Geometry: final body of the model. Coordinates: model frame, mm. A direction names the side the tool comes from. Round coordinates to 2 decimals unless told otherwise and drop trailing zeros. Loops run counter-clockwise (first coordinate to the right, second up) from the corner with the lowest first, then second, coordinate; pieces in that order, holes last. Notation, with made-up numbers: (-37.75, 76) - (9.25, 76) arc R23 ccw to (9.25, 85) - close; hole circle Ø9 at (11, 16). An arc over 180 degrees is marked (long way). Use CSV: the item, a comma, the result in double quotes.
from build123d import *

# Parameters (mm, degrees)
SKETCH1_R                              = 175
BOSS_EXTRUDE1_DEPTH                    = 30
CSK_FOR_M10_SFHCS1_D                   = 11
CSK_FOR_M10_SFHCS1_CSINK_D             = 22.4
CSK_FOR_M10_SFHCS1_CSINK_ANGLE         = 90
F_6_0MM_DOWEL_HOLE1_D                  = 6
CUT_EXTRUDE2_DEPTH                     = 10
TAP_DRILL_FOR_M12X1_75_TAP1_AT_2_COUNT = 2
TAP_DRILL_FOR_M12X1_75_TAP1_AT_2_PITCH = 116
TAP_DRILL_FOR_M12X1_75_TAP1_AT_3_COUNT = 2
TAP_DRILL_FOR_M12X1_75_TAP1_AT_3_PITCH = 257.596583828
TAP_DRILL_FOR_M12X1_75_TAP1_AT_4_COUNT = 2
TAP_DRILL_FOR_M12X1_75_TAP1_AT_4_PITCH = 230


with BuildPart() as part:
    # Sketch1 → Boss-Extrude1 (new body)
    with BuildSketch(Plane(origin=(0, 0, 0), x_dir=(1, 0, 0), z_dir=(0, 1, 0))):
        Circle(SKETCH1_R)
    extrude(amount=BOSS_EXTRUDE1_DEPTH)

    # CSK for M10 SFHCS1 (through all)
    with Locations(Plane(origin=(0, 30, 0), x_dir=(1, 0, 0), z_dir=(0, 1, 0))):
        with Locations((-150, 0), (0, -150), (150, 0), (0, 150)):
            CounterSinkHole(CSK_FOR_M10_SFHCS1_D / 2, CSK_FOR_M10_SFHCS1_CSINK_D / 2, counter_sink_angle=CSK_FOR_M10_SFHCS1_CSINK_ANGLE)

    # Ø6.0mm Dowel Hole1 (through all)
    with Locations(Plane(origin=(0, 30, 0), x_dir=(1, 0, 0), z_dir=(0, 1, 0))):
        with Locations((-97.227182413, -97.227182413), (97.227182413, -97.227182413), (97.227182413, 97.227182413), (-97.227182413, 97.227182413)):
            Hole(F_6_0MM_DOWEL_HOLE1_D / 2)

    # Sketch14 → Cut-Extrude2 (cut)
    with BuildSketch(Plane(origin=(0, 30, 0), x_dir=(1, 0, 0), z_dir=(0, 1, 0))):
        with BuildLine():
            Line((-74, -40), (74, -40))
            ThreePointArc((74, -40), (78.242640687, -41.757359313), (80, -46))
            Line((80, -46), (80, -84))
            ThreePointArc((80, -84), (78.242640687, -88.242640687), (74, -90))
            Line((74, -90), (-74, -90))
            ThreePointArc((-74, -90), (-78.242640687, -88.242640687), (-80, -84))
            Line((-80, -84), (-80, -46))
            ThreePointArc((-80, -46), (-78.242640687, -41.757359313), (-74, -40))
        make_face()
        with BuildLine():
            Line((80, 46), (80, 84))
            ThreePointArc((80, 84), (78.242640687, 88.242640687), (74, 90))
            Line((74, 90), (-74, 90))
            ThreePointArc((-74, 90), (-78.242640687, 88.242640687), (-80, 84))
            Line((-80, 84), (-80, 46))
            ThreePointArc((-80, 46), (-78.242640687, 41.757359313), (-74, 40))
            Line((-74, 40), (74, 40))
            ThreePointArc((74, 40), (78.242640687, 41.757359313), (80, 46))
        make_face()
    extrude(amount=-CUT_EXTRUDE2_DEPTH, mode=Mode.SUBTRACT)

    # Sketch21 → Tap Drill for M12x1.75 Tap1 (revolve, cut)
    with BuildSketch(Plane(origin=(-58, 30, -115), x_dir=(0, 0, 1), z_dir=(1, 0, 0))):
        Polygon((0, 0), (0, 30), (12.5, 30), (5.1, 19.43170475), (5.1, 0), align=None)
    tap_drill_for_m12x1_75_tap1 = revolve(axis=Axis((-58, 36.35, -115), (0, -1, 0)), mode=Mode.SUBTRACT)

    # Tap Drill for M12x1.75 Tap1 at 2: Tap Drill for M12x1.75 Tap1 ×2
    with Locations(*[(i * TAP_DRILL_FOR_M12X1_75_TAP1_AT_2_PITCH, 0, 0) for i in range(1, TAP_DRILL_FOR_M12X1_75_TAP1_AT_2_COUNT)]):
        add(tap_drill_for_m12x1_75_tap1, mode=Mode.SUBTRACT)

    # Tap Drill for M12x1.75 Tap1 at 3: Tap Drill for M12x1.75 Tap1 ×2
    with Locations(*[Vector(0.450316531, 0, 0.892868984) * (i * TAP_DRILL_FOR_M12X1_75_TAP1_AT_3_PITCH) for i in range(1, TAP_DRILL_FOR_M12X1_75_TAP1_AT_3_COUNT)]):
        add(tap_drill_for_m12x1_75_tap1, mode=Mode.SUBTRACT)

    # Tap Drill for M12x1.75 Tap1 at 4: Tap Drill for M12x1.75 Tap1 ×2
    with Locations(*[(0, 0, i * TAP_DRILL_FOR_M12X1_75_TAP1_AT_4_PITCH) for i in range(1, TAP_DRILL_FOR_M12X1_75_TAP1_AT_4_COUNT)]):
        add(tap_drill_for_m12x1_75_tap1, mode=Mode.SUBTRACT)


solid = part.part
Item 1: Section A-A on x = 0. Return the cut outline in (y, z), plus the area to 4 significant figures.
Final values:
outline,"(0, -175) - (30, -175) - (30, -161.2) - (24.3, -155.5) - (0, -155.5) - close; (0, -144.5) - (24.3, -144.5) - (30, -138.8) - (30, -90) - (20, -90) - (20, -40) - (30, -40) - (30, 40) - (20, 40) - (20, 90) - (30, 90) - (30, 138.8) - (24.3, 144.5) - (0, 144.5) - close; (0, 155.5) - (24.3, 155.5) - (30, 161.2) - (30, 175) - (0, 175) - close"
area,"8,775 mm²"
Item 2: Pin query (flat end, axial travel): P1, Ø3, axis at x = -17.5, y = 26, coming from the -Z side; P2, Ø8, axis at x = -97.23, z = 97.23, coming from the -Y side; P3, Ø13.5, axis at x = 58, z = -115, coming from the -Y side; P4, Ø17.5, axis at x = 0, z = -150, coming from the +Y side. Return the tip coordinate at first contact, or that it passes through.
Final values:
P1,"stops at z = -174.27"
P2,"stops at y = 0"
P3,"stops at y = 8.21"
P4,"stops at y = 27.55"
Item 3: Mould query, pull axis X, two halves, no side actions, for faces 3 (the cylindrical face through (-128.982, 14.79, -118.273)), 4 (the flat face through (-2, 0, -2)), 5 (the cylindrical face through (-61.4, 20.4, 111.2)). Classes: released by +X, released by -X, zero draft, split by the parting line, or undercut.
Final values:
face 3,"split by the parting line"
face 4,"zero draft"
face 5,"undercut"
Item 4: Material intervals for line 1 (Z direction, x = -61, y = 6); line 2 (Z direction, x = -58, y = 21.25); line 3 (Z direction, x = -58, y = 17.5), sorted ascending.
Final values:
line 1,"z = -164.02 to -122.74, -107.26 to 107.26, 122.74 to 164.02"
line 2,"z = -165.11 to -120.1, -109.9 to -90, -40 to 40, 90 to 109.9, 120.1 to 165.11"
line 3,"z = -165.11 to -120.1, -109.9 to 109.9, 120.1 to 165.11"
Item 5: Section C-C on z = 150. Return the cut outline in (x, y), plus the area to 3 significant figures.
Final values:
outline,"(-90.14, 0) - (-5.5, 0) - (-5.5, 24.3) - (-11.2, 30) - (-90.14, 30) - close; (5.5, 0) - (90.14, 0) - (90.14, 30) - (11.2, 30) - (5.5, 24.3) - close"
area,"5,050 mm²"
Item 6: Section B-B on z = 0. Return the cut outline in (x, y), plus the area to 4 significant figures.
Final values:
outline,"(-175, 0) - (-155.5, 0) - (-155.5, 24.3) - (-161.2, 30) - (-175, 30) - close; (-144.5, 0) - (144.5, 0) - (144.5, 24.3) - (138.8, 30) - (-138.8, 30) - (-144.5, 24.3) - close; (155.5, 0) - (175, 0) - (175, 30) - (161.2, 30) - (155.5, 24.3) - close"
area,"9,775 mm²"
Item 7: Section D-D on x = 150. Return the cut outline in (y, z), plus the area to 3 significant figures.
Final values:
outline,"(0, -90.14) - (30, -90.14) - (30, -11.2) - (24.3, -5.5) - (0, -5.5) - close; (0, 5.5) - (24.3, 5.5) - (30, 11.2) - (30, 90.14) - (0, 90.14) - close"
area,"5,050 mm²"
Item 8: Reachability of faces 1 (the conical face through (-58.24, 10.06, 109.55)), 2 (the flat face through (-80, 25, 65)) from +Z, -Z, +X, -X, +Y, -Y: full face, straight path, thin tool, end or side. Return the list, or none.
Final values:
face 1,"-Y"
face 2,"+Y"
